Source: CAD feature listing. Evaluate the final solid. Frame: model axes, mm. A direction names the side the tool comes from. Coordinates: 2 decimals unless noted, no trailing zeros. Write each loop counter-clockwise with the first axis right and the second up, starting at its lowest first coordinate (ties: lowest second). Pieces come first, ordered by that corner, then holes. Notation, with made-up numbers: M 35,25 L 87,25 A25 cw 87,59 Z; hole C 84,33 d1. An arc over 180 degrees is marked long. Answer as CSV lines item,"result". Start each with the question number.
1. Line query: probe 1 along X at (y, z) = (20.75, 0); probe 2 along Y at (x, z) = (9.5, -1.75); probe 3 along X at (y, z) = (7, 0). Output: solid intervals per line, ascending. Write a range as [from, to].
2. Section A-A on z = 0. Return the cut outline in (x, y), plus the area to 3 significant figures.
3. Section D-D on x = 14. Return the cut outline in (y, z).
4. Mould query, pull axis X, two halves, no side actions, for faces 4 (the face through (9.6, 2, 1)), 5 (the face through (-2.5, 10.8, -0.1)), 6 (the face through (-1, 11, 0)), 7 (the face through (14.613, 1.493, -0.325)). Classes: pulls with the +X half, pulls with the -X half, needs draft (parallel to the pull), parting line crosses it, or undercut.
5. Reachability of faces 1 (the face through (7.134, 10.888, 0.024)), 2 (the face through (12, 1, 0)), 3 (the face through (6, 22, 0)) from +Z, -Z, +X, -X, +Y, -Y: full face, straight path, thin tool, end or side. Return the list, or none.
6. Section B-B on y = 18.25. Return the cut outline in (x, z), plus the area to 3 significant figures.
7. Section C-C on x = 9.25. Return the cut outline in (y, z), plus the area to 3 significant figures.
8. Contact query for flat-ended pins moving along their axis: pin 1 Ø3 at (x, z) = (12.13, 0) entering from +Y; pin 2 Ø1.5 at (y, z) = (8.5, -2) entering from -X; pin 3 Ø2 at (x, y) = (8, 5.5) entering from -Z. Output: stop coordinate, or through.
```python
from build123d import *

# Parameters (mm, degrees)
SKETCH1_R               = 1
SKETCH1_R_2             = 2.5
BOSS_EXTRUDE5_DEPTH     = 2
SKETCH1_7_R             = 2.5
SKETCH1_7_R_2           = 1
BOSS_EXTRUDE6_DEPTH     = 22
BOSS_EXTRUDE7_START     = 20
BOSS_EXTRUDE7_OUTLINE_R = 2.5
BOSS_EXTRUDE7_DEPTH     = 2
SKETCH1_9_R             = 2.5
BOSS_EXTRUDE8_DEPTH     = 1
FILLET3_R               = 1
FILLET1_R               = 1


# Read off the part's stored shape, not the designer's step: Boss-Extrude7
with BuildPart() as part:
    # Sketch1 → Boss-Extrude5 (new body)
    with BuildSketch(Plane(origin=(0, 0, 0), x_dir=(1, 0, 0), z_dir=(0, 1, 0))):
        with BuildLine():
            ThreePointArc((-0.206033327, 2.491495589), (-2.5, 0), (-0.206033327, -2.491495589))
            Line((-0.206033327, -2.491495589), (11.845512634, -3.488093824))
            ThreePointArc((11.845512634, -3.488093824), (15.633959292, 0), (11.845512634, 3.488093824))
            Line((11.845512634, 3.488093824), (-0.206033327, 2.491495589))
        make_face()
        with Locations(Location((0, 0, 0), (0, 0, 270))):
            Circle(SKETCH1_R, mode=Mode.SUBTRACT)
        with Locations(Location((12.133959292, 0, 0), (0, 0, 270))):
            Circle(SKETCH1_R_2, mode=Mode.SUBTRACT)
    extrude(amount=BOSS_EXTRUDE5_DEPTH)

    # Sketch1<7> → Boss-Extrude6 (add)
    # profile 1 of 2: a face of its own
    with BuildSketch(Plane(origin=(0, 0, 0), x_dir=(1, 0, 0), z_dir=(0, 1, 0))):
        Circle(SKETCH1_7_R)
        with Locations(Location((0, 0, 0), (0, 0, 270))):
            Circle(SKETCH1_7_R_2, mode=Mode.SUBTRACT)
    # profile 2 of 2: a face of its own
    with BuildSketch(Plane(origin=(0, 0, 0), x_dir=(1, 0, 0), z_dir=(0, 1, 0))):
        with BuildLine():
            Line((8.286945149, 3.193819373), (-0.206033327, 2.491495589))
            ThreePointArc((-0.206033327, 2.491495589), (1.693357122, 1.839168741), (2.5, 0))
            ThreePointArc((2.5, 0), (1.693357122, -1.839168741), (-0.206033327, -2.491495589))
            Line((-0.206033327, -2.491495589), (8.286945149, -3.193819373))
            ThreePointArc((8.286945149, -3.193819373), (7.133959292, 0), (8.286945149, 3.193819373))
        make_face()
    extrude(amount=BOSS_EXTRUDE6_DEPTH)

    # Boss-Extrude7 outline → Boss-Extrude7 (add)
    with BuildSketch(Plane(origin=(0, 0, 0), x_dir=(1, 0, 0), z_dir=(0, 1, 0)).offset(BOSS_EXTRUDE7_START)):
        with BuildLine():
            Line((8.286945149, -3.193819373), (11.845512634, -3.488093824))
            ThreePointArc((11.845512634, -3.488093824), (15.633959292, 0), (11.845512634, 3.488093824))
            Line((11.845512634, 3.488093824), (8.286945149, 3.193819373))
            ThreePointArc((8.286945149, 3.193819373), (7.133959292, 0), (8.286945149, -3.193819373))
        make_face()
        with Locations((12.133959292, 0)):
            Circle(BOSS_EXTRUDE7_OUTLINE_R, mode=Mode.SUBTRACT)
    extrude(amount=BOSS_EXTRUDE7_DEPTH)

    # Sketch1<9> → Boss-Extrude8 (add)
    with BuildSketch(Plane(origin=(0, 0, 0), x_dir=(1, 0, 0), z_dir=(0, 1, 0))):
        with Locations(Location((12.133959292, 0, 0), (0, 0, 270))):
            Circle(SKETCH1_9_R)
    extrude(amount=BOSS_EXTRUDE8_DEPTH)

    # Fillet3
    # the kernel refuses this fillet: 1 mm, written as the material it takes off along each edge
    with BuildSketch(Plane(origin=(8.286945149, 2, 3.193819373), x_dir=(-0.49694917619000334, 0, -0.8677796473091985), z_dir=(0, 1, 0))) as fillet3_piece_1:
        with BuildLine():
            CenterArc((1.891474067, 0.985105296), FILLET3_R, 145.474338823, 114.624318352)
            Line((1.067601639, 1.55188058), (0, 0))
            ThreePointArc((0, 0), (0.85976094, 0.074473518), (1.719521879, 0))
        make_face()
    extrude(amount=18, mode=Mode.SUBTRACT)
    with BuildSketch(Plane(origin=(8.286945149, 2, -3.193819373), x_dir=(-0.9965982354592262, 0, 0.08241333071510189), z_dir=(0, 1, 0))) as fillet3_piece_2:
        with BuildLine():
            CenterArc((1.883641843, 1), FILLET3_R, 155.375681648, 114.624318352)
            ThreePointArc((0.9745825, 1.416666667), (0.548647928, 0.666123584), (0, 0))
            Line((0, 0), (1.883641843, 0))
        make_face()
    extrude(amount=18, mode=Mode.SUBTRACT)

    # Fillet1
    # the kernel refuses this fillet: 1 mm, written as the material it adds along each edge
    with BuildSketch(Plane(origin=(12.133959294, 20, 0), x_dir=(-0.9403058248886403, 0, -0.34033065639241744), z_dir=(0.34033065639241744, 0, -0.9403058248886403))) as fillet1_piece_1:
        with BuildLine():
            CenterArc((5.000000002 - FILLET1_R, -FILLET1_R), FILLET1_R, 0, 90)
            Line((5.000000002 - FILLET1_R, 0), (5.000000002, 0))
            Line((5.000000002, 0), (5.000000002, -FILLET1_R))
        make_face()
    revolve(axis=Axis((12.133959294, 20, 0), (0, 1, 0)), revolution_arc=39.794041437)
    with BuildSketch(Plane(origin=(12.133959292, 2, 0), x_dir=(-0.9403058248462457, 0, 0.3403306565095503), z_dir=(0.3403306565095503, 0, 0.9403058248462457))) as fillet1_piece_2:
        with BuildLine():
            CenterArc((5 - FILLET1_R, -FILLET1_R), FILLET1_R, 0, 90)
            Line((5 - FILLET1_R, 0), (5, 0))
            Line((5, 0), (5, -FILLET1_R))
        make_face()
    revolve(axis=Axis((12.133959292, 2, 0), (0, -1, 0)), revolution_arc=39.794041451)
    with BuildSketch(Plane(origin=(6.492124343, 2, -2.041983939), x_dir=(0.9403058248461986, 0, 0.34033065650968036), z_dir=(-0.34033065650968036, 0, 0.9403058248461986))) as fillet1_piece_3_section:
        with BuildLine():
            CenterArc((1 + FILLET1_R, FILLET1_R), FILLET1_R, 180, 90)
            Line((1 + FILLET1_R, 0), (1, 0))
            Line((1, 0), (1, FILLET1_R))
        make_face()
    fillet1_piece_3 = revolve(axis=Axis((6.492124343, 2, -2.041983939), (0, 1, 0)), revolution_arc=257.957117876, mode=Mode.PRIVATE)
    fillet1_piece_3 = split(fillet1_piece_3, bisect_by=Plane(origin=(7.34883742, 2.262262875, -3.116242893), z_dir=(0.08241333071510651, 0, 0.9965982354592259)), keep=Keep.TOP, mode=Mode.PRIVATE)
    add(fillet1_piece_3)
    with BuildSketch(Plane(origin=(6.492124343, 20, -2.041983939), x_dir=(0.9403058248461986, 0, 0.34033065650968036), z_dir=(-0.34033065650968036, 0, 0.9403058248461986))) as fillet1_piece_4_section:
        with BuildLine():
            CenterArc((1 + FILLET1_R, -FILLET1_R), FILLET1_R, 90, 90)
            Line((1, -FILLET1_R), (1, 0))
            Line((1, 0), (1 + FILLET1_R, 0))
        make_face()
    fillet1_piece_4 = revolve(axis=Axis((6.492124343, 20, -2.041983939), (0, 1, 0)), revolution_arc=257.957117876, mode=Mode.PRIVATE)
    fillet1_piece_4 = split(fillet1_piece_4, bisect_by=Plane(origin=(7.693506276, 19.839747829, -3.14474516), z_dir=(0.08241333071510651, 0, 0.9965982354592259)), keep=Keep.TOP, mode=Mode.PRIVATE)
    add(fillet1_piece_4)
    with BuildSketch(Plane(origin=(6.492124343, 2, 2.041983939), x_dir=(-0.5290294610510079, 0, -0.8486034582418812), z_dir=(0.8486034582418812, 0, -0.5290294610510079))) as fillet1_piece_5_section:
        with BuildLine():
            CenterArc((1 + FILLET1_R, FILLET1_R), FILLET1_R, 180, 90)
            Line((1 + FILLET1_R, 0), (1, 0))
            Line((1, 0), (1, FILLET1_R))
        make_face()
    fillet1_piece_5 = revolve(axis=Axis((6.492124343, 2, 2.041983939), (0, 1, 0)), revolution_arc=257.957117876, mode=Mode.PRIVATE)
    fillet1_piece_5 = split(fillet1_piece_5, bisect_by=Plane(origin=(7.348749187, 2.26222623, 3.116235597), z_dir=(0.08241333071510651, 0, -0.9965982354592259)), keep=Keep.TOP, mode=Mode.PRIVATE)
    add(fillet1_piece_5)
    with BuildSketch(Plane(origin=(6.492124343, 20, 2.041983939), x_dir=(-0.5290294610510079, 0, -0.8486034582418812), z_dir=(0.8486034582418812, 0, -0.5290294610510079))) as fillet1_piece_6_section:
        with BuildLine():
            CenterArc((1 + FILLET1_R, -FILLET1_R), FILLET1_R, 90, 90)
            Line((1 + FILLET1_R, 0), (1, 0))
            Line((1, 0), (1, -FILLET1_R))
        make_face()
    fillet1_piece_6 = revolve(axis=Axis((6.492124343, 20, 2.041983939), (0, 1, 0)), revolution_arc=257.957117876, mode=Mode.PRIVATE)
    fillet1_piece_6 = split(fillet1_piece_6, bisect_by=Plane(origin=(7.34874918, 19.737773776, 3.116235596), z_dir=(0.08241333071510651, 0, -0.9965982354592259)), keep=Keep.TOP, mode=Mode.PRIVATE)
    add(fillet1_piece_6)


solid = part.part
```
Values:
1,probe 1,"[-2.5, -1], [1, 9.63], [14.63, 15.63]"
1,probe 2,"[0, 2], [20, 22]"
1,probe 3,"[-2.5, -1], [1, 7.13]"
2,outline,"M -2.5,0 L -1,0 L -1,22 L -2.5,22 Z; M 1,0 L 15.63,0 L 15.63,2 L 14.63,2 L 14.63,1 L 9.63,1 L 9.63,2 L 8.13,2 A1 cw 7.13,3 L 7.13,19 A1 cw 8.13,20 L 9.63,20 L 9.63,22 L 1,22 Z; M 14.63,20 L 15.63,20 L 15.63,22 L 14.63,22 Z"
2,area,"187 mm²"
3,outline,"M 0,-2.96 L 2,-2.96 L 2,-1.66 L 1,-1.66 L 1,1.66 L 2,1.66 L 2,2.96 L 0,2.96 Z; M 20,-2.96 L 22,-2.96 L 22,-1.66 L 20,-1.66 Z; M 20,1.66 L 22,1.66 L 22,2.96 L 20,2.96 Z"
4,face 4,"needs draft"
4,face 5,"pulls with the -X half"
4,face 6,"undercut"
4,face 7,"undercut"
5,face 1,"+X"
5,face 2,"+Y"
5,face 3,"+Z, -Z, +X, -X, +Y"
6,outline,"M -0.21,-2.49 L 6.41,-3.04 A1 ccw 7.43,-1.7 A5 cw 7.43,1.7 A1 ccw 6.41,3.04 L -0.21,2.49 A2.5 ccw Z; hole C 0,0 d2"
6,area,"47.5 mm²"
7,outline,"M 0,-3.27 L 2,-3.27 L 2,3.27 L 0,3.27 Z; M 20,-3.27 L 22,-3.27 L 22,3.27 L 20,3.27 Z"
7,area,"26.2 mm²"
8,pin 1,"y = 1"
8,pin 2,"x = -2.17"
8,pin 3,"z = -2.9"
